Source: CAD feature listing. Evaluate the final solid. Frame: model axes, mm. Face numbers are marked on the shaded views. A direction names the side the tool comes from. Round coordinates to 2 decimals unless told otherwise and drop trailing zeros. Order: outer loops, then holes, each group sorted by start corner. A loop starts at its lowest first (then second) coordinate and runs counter-clockwise, first axis right, second up.
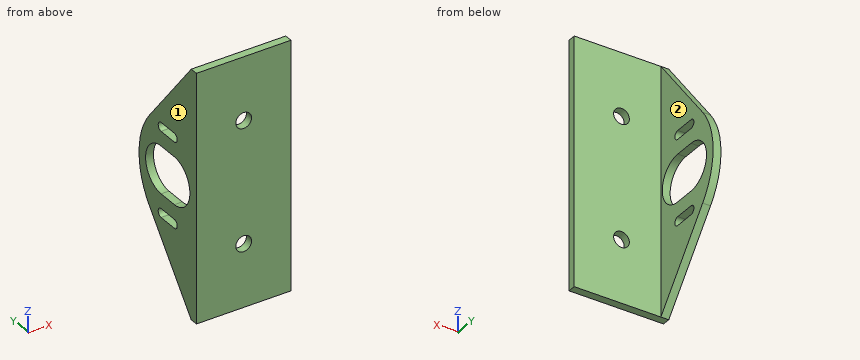
```python
from build123d import *

# Parameters (mm, degrees)
SKETCH1_W           = 133.35
SKETCH1_H           = 50.8
BOSS_EXTRUDE1_DEPTH = 3.175
SKETCH4_W           = 76.2
SKETCH4_H           = 3.175
BOSS_EXTRUDE2_DEPTH = 147.32
SKETCH3_R           = 3.175
CUT_EXTRUDE2_DEPTH  = 4.175
SKETCH5_W           = 133.35
SKETCH5_H           = 88.9
CUT_EXTRUDE3_DEPTH  = 4.175
SKETCH7_W           = 22.225
SKETCH7_H           = 109.22
CUT_EXTRUDE4_DEPTH  = 4.175
SKETCH8_OUTSIDE_W   = 80.349
SKETCH8_OUTSIDE_H   = 135.594
SKETCH8_OUTSIDE_W_2 = 47.625
SKETCH8_OUTSIDE_H_2 = 99.906666667
CUT_EXTRUDE5_DEPTH  = 4.175
BOSS_EXTRUDE4_DEPTH = 3.175
SKETCH10_W          = 12.7
SKETCH10_H          = 99.906666667
CUT_EXTRUDE6_DEPTH  = 4.175
CUT_EXTRUDE7_DEPTH  = 39.1


with BuildPart() as part:
    # Sketch1 → Boss-Extrude1 (new body)
    with BuildSketch(Plane(origin=(0, 0, 0), x_dir=(1, 0, 0), z_dir=(0, 1, 0))):
        Rectangle(SKETCH1_W, SKETCH1_H)
    extrude(amount=BOSS_EXTRUDE1_DEPTH)

    # Sketch4 → Boss-Extrude2 (add)
    with BuildSketch(Plane.XY.offset(25.4)):
        with Locations((0, 1.5875)):
            Rectangle(SKETCH4_W, SKETCH4_H)
    extrude(amount=BOSS_EXTRUDE2_DEPTH)

    # Sketch3 → Cut-Extrude2 (cut, through all)
    with BuildSketch(Plane(origin=(0, 3.175, 0), x_dir=(1, 0, 0), z_dir=(0, 1, 0))):
        Circle(SKETCH3_R)
        with Locations((0, -49.106666667)):
            Circle(SKETCH3_R)
        with Locations((0, -98.213333333)):
            Circle(SKETCH3_R)
        with Locations((0, -147.32)):
            Circle(SKETCH3_R)
    extrude(amount=-CUT_EXTRUDE2_DEPTH, mode=Mode.SUBTRACT)

    # Sketch5 → Cut-Extrude3 (cut, through all)
    with BuildSketch(Plane(origin=(0, 3.175, 0), x_dir=(1, 0, 0), z_dir=(0, 1, 0))):
        with Locations((0, -19.05)):
            Rectangle(SKETCH5_W, SKETCH5_H)
    extrude(amount=-CUT_EXTRUDE3_DEPTH, mode=Mode.SUBTRACT)

    # Sketch7 → Cut-Extrude4 (cut, through all)
    with BuildSketch(Plane(origin=(0, 3.175, 0), x_dir=(1, 0, 0), z_dir=(0, 1, 0))):
        with Locations((-26.9875, -118.11)):
            Rectangle(SKETCH7_W, SKETCH7_H)
    extrude(amount=-CUT_EXTRUDE4_DEPTH, mode=Mode.SUBTRACT)

    # Sketch8 outside → Cut-Extrude5 (cut, through all)
    with BuildSketch(Plane(origin=(0, 3.175, 0), x_dir=(1, 0, 0), z_dir=(0, 1, 0))):
        with Locations((11.1125, -118.11)):
            Rectangle(SKETCH8_OUTSIDE_W, SKETCH8_OUTSIDE_H)
        with Locations((7.9375, -122.766666667)):
            Rectangle(SKETCH8_OUTSIDE_W_2, SKETCH8_OUTSIDE_H_2, mode=Mode.SUBTRACT)
    extrude(amount=-CUT_EXTRUDE5_DEPTH, mode=Mode.SUBTRACT)

    # Sketch9 → Boss-Extrude4 (add)
    with BuildSketch(Plane.ZY.offset(15.875)):
        with BuildLine():
            Line((172.72, 3.175), (140.847432308, 28.849821314))
            ThreePointArc((140.847432308, 28.849821314), (122.766666667, 35.226473065), (104.685901025, 28.849821314))
            Line((104.685901025, 28.849821314), (72.813333333, 3.175))
            Line((72.813333333, 3.175), (72.813333333, 0))
            Line((72.813333333, 0), (172.72, 0))
            Line((172.72, 0), (172.72, 3.175))
        make_face()
    extrude(amount=BOSS_EXTRUDE4_DEPTH)

    # Sketch10 → Cut-Extrude6 (cut, through all)
    with BuildSketch(Plane(origin=(0, 3.175, 0), x_dir=(1, 0, 0), z_dir=(0, 1, 0))):
        with Locations((25.4, -122.766666667)):
            Rectangle(SKETCH10_W, SKETCH10_H)
    extrude(amount=-CUT_EXTRUDE6_DEPTH, mode=Mode.SUBTRACT)

    # Sketch11 → Cut-Extrude7 (cut, through all)
    with BuildSketch(Plane.ZY.offset(19.05)):
        with BuildLine():
            Line((132.291666667, 21.680516849), (132.291666667, 13.545956216))
            ThreePointArc((132.291666667, 13.545956216), (122.766666667, 4.020956216), (113.241666667, 13.545956216))
            Line((113.241666667, 13.545956216), (113.241666667, 21.680516849))
            ThreePointArc((113.241666667, 21.680516849), (122.766666667, 31.205516849), (132.291666667, 21.680516849))
        make_face()
        with BuildLine():
            Line((141.71638956, 21.680516849), (141.71638956, 13.545956216))
            ThreePointArc((141.71638956, 13.545956216), (139.93838956, 11.767956216), (138.16038956, 13.545956216))
            Line((138.16038956, 13.545956216), (138.16038956, 21.680516849))
            ThreePointArc((138.16038956, 21.680516849), (139.93838956, 23.458516849), (141.71638956, 21.680516849))
        make_face()
        with BuildLine():
            Line((107.372943773, 21.680516849), (107.372943773, 13.545956216))
            ThreePointArc((107.372943773, 13.545956216), (105.594943773, 11.767956216), (103.816943773, 13.545956216))
            Line((103.816943773, 13.545956216), (103.816943773, 21.680516849))
            ThreePointArc((103.816943773, 21.680516849), (105.594943773, 23.458516849), (107.372943773, 21.680516849))
        make_face()
    extrude(amount=-CUT_EXTRUDE7_DEPTH, mode=Mode.SUBTRACT)


solid = part.part
```
1. First-contact query: pin 1 (8 mm diameter, centred on x = 6.5, z = 150.5, fed in from +Y) (3 decimals); pin 2 (4 mm diameter, centred on x = 0, z = 98.21, fed in from -Y); pin 3 (3.5 mm diameter, centred on x = -17.5, y = 17, fed in from -Z); pin 4 (2.5 mm diameter, centred on x = -17.5, y = 17.5, fed in from +Z). Flat tips, straight axial feed; report the tip coordinate or a pass-through.
2. Section A-A on x = 0. Return loops of the section in (y, z) (3 decimals), plus the area to 3 significant figures.
3. Section B-B on y = 15. Return loops of the section in (x, z) (3 decimals), plus the area to 3 significant figures.
4. Section D-D on y = 26. Return loops of the section in (x, z) (3 decimals).
5. Line query: line 1 along Z through (x, y) = (0, 2.1) (3 decimals); line 2 along X through (y, z) = (1.1, 147.32) (3 decimals); line 3 along X through (y, z) = (6.5, 132) (3 decimals). Output: solid intervals per line, ascending.
6. Section C-C on z = 148.5. Return loops of the section in (x, y) (3 decimals).
7. Access query for the marked faces 1 and 2. Directions: +Z, -Z, +X, -X, +Y, -Y. A direction counts if a zero-diameter tool reaches every point of the face in a straight line with its end or side. Return the directions, or none.
Result:
1. pin 1: stops at y = 3.175
1. pin 2: passes through
1. pin 3: stops at z = 87.8
1. pin 4: stops at z = 156.49
2. outline: (0, 72.813) - (3.175, 72.813) - (3.175, 95.038) - (0, 95.038) - close; (0, 101.388) - (3.175, 101.388) - (3.175, 144.145) - (0, 144.145) - close; (0, 150.495) - (3.175, 150.495) - (3.175, 172.72) - (0, 172.72) - close
2. area: 277 mm2
3. outline: (-19.05, 87.493) - (-15.875, 87.493) - (-15.875, 103.817) - (-19.05, 103.817) - close; (-19.05, 107.373) - (-15.875, 107.373) - (-15.875, 113.242) - (-19.05, 113.242) - close; (-19.05, 132.292) - (-15.875, 132.292) - (-15.875, 138.16) - (-19.05, 138.16) - close; (-19.05, 141.716) - (-15.875, 141.716) - (-15.875, 158.041) - (-19.05, 158.041) - close
3. area: 141 mm2
4. outline: (-19.05, 101.148) - (-15.875, 101.148) - (-15.875, 114.277) - (-19.05, 114.277) - close; (-19.05, 131.256) - (-15.875, 131.256) - (-15.875, 144.385) - (-19.05, 144.385) - close
5. line 1: z = 72.813 to 95.038, 101.388 to 144.145, 150.495 to 172.72
5. line 2: x = -19.05 to -3.175, 3.175 to 19.05
5. line 3: x = -19.05 to -15.875
6. outline: (-19.05, 0) - (-2.948, 0) - (-2.948, 3.175) - (-15.875, 3.175) - (-15.875, 22.685) - (-19.05, 22.685) - close; (2.948, 0) - (19.05, 0) - (19.05, 3.175) - (2.948, 3.175) - close
7. face 1: +Z, -Z, -X, +Y, -Y
7. face 2: +Z, -Z, +X, +Y
